```python
from build123d import *

# Parameters (mm, degrees)
SKETCH1_R          = 12.573
EXTRUDE1_DEPTH     = 2.1844
CUT_EXTRUDE1_DEPTH = 18.914582366
SKETCH4_R          = 4.6101
CUT_EXTRUDE2_DEPTH = 18.914582366
SKETCH5_R          = 0.508
CUT_EXTRUDE3_DEPTH = 18.914582366


with BuildPart() as part:
    # Sketch1 → Extrude1 (new body)
    with BuildSketch(Plane.XY):
        Circle(SKETCH1_R)
    extrude(amount=EXTRUDE1_DEPTH)

    # Sketch2 → Cut-Extrude1 (cut, through all)
    with BuildSketch(Plane.XY.offset(2.1844)):
        with BuildLine():
            Line((-7.159213379, 8.746626366), (-7.963619377, 9.729393373))
            ThreePointArc((-7.963619377, 9.729393373), (-8.89045356, 8.89045356), (-9.729393373, 7.963619377))
            Line((-9.729393373, 7.963619377), (-8.746626366, 7.159213379))
            ThreePointArc((-8.746626366, 7.159213379), (-9.076228299, 6.736459669), (-9.385415604, 6.298554036))
            Line((-9.385415604, 6.298554036), (-5.244666377, 3.907891355))
            ThreePointArc((-5.244666377, 3.907891355), (-4.624831902, 4.624831902), (-3.907891355, 5.244666377))
            Line((-3.907891355, 5.244666377), (-6.298554036, 9.385415604))
            ThreePointArc((-6.298554036, 9.385415604), (-6.736459669, 9.076228299), (-7.159213379, 8.746626366))
        make_face()
        with BuildLine():
            Line((-10.573373841, 3.995193941), (-11.761393373, 4.444092136))
            ThreePointArc((-11.761393373, 4.444092136), (-12.144585414, 3.254131854), (-12.407711513, 2.032))
            Line((-12.407711513, 2.032), (-11.15440732, 1.826747475))
            ThreePointArc((-11.15440732, 1.826747475), (-11.228474112, 1.295831056), (-11.277285356, 0.762))
            Line((-11.277285356, 0.762), (-6.495959994, 0.762))
            ThreePointArc((-6.495959994, 0.762), (-6.317637867, 1.692805964), (-6.006666377, 2.58806864))
            Line((-6.006666377, 2.58806864), (-10.147415604, 4.97873132))
            ThreePointArc((-10.147415604, 4.97873132), (-10.372059354, 4.492014443), (-10.573373841, 3.995193941))
        make_face()
        with BuildLine():
            Line((-11.15440732, -1.826747475), (-12.407711513, -2.032))
            ThreePointArc((-12.407711513, -2.032), (-12.144585414, -3.254131854), (-11.761393373, -4.444092136))
            Line((-11.761393373, -4.444092136), (-10.573373841, -3.995193941))
            ThreePointArc((-10.573373841, -3.995193941), (-10.372059354, -4.492014443), (-10.147415604, -4.97873132))
            Line((-10.147415604, -4.97873132), (-6.006666377, -2.58806864))
            ThreePointArc((-6.006666377, -2.58806864), (-6.317637867, -1.692805964), (-6.495959994, -0.762))
            Line((-6.495959994, -0.762), (-11.277285356, -0.762))
            ThreePointArc((-11.277285356, -0.762), (-11.228474112, -1.295831056), (-11.15440732, -1.826747475))
        make_face()
        with BuildLine():
            Line((-8.746626366, -7.159213379), (-9.729393373, -7.963619377))
            ThreePointArc((-9.729393373, -7.963619377), (-8.89045356, -8.89045356), (-7.963619377, -9.729393373))
            Line((-7.963619377, -9.729393373), (-7.159213379, -8.746626366))
            ThreePointArc((-7.159213379, -8.746626366), (-6.736459669, -9.076228299), (-6.298554036, -9.385415604))
            Line((-6.298554036, -9.385415604), (-3.907891355, -5.244666377))
            ThreePointArc((-3.907891355, -5.244666377), (-4.624831902, -4.624831902), (-5.244666377, -3.907891355))
            Line((-5.244666377, -3.907891355), (-9.385415604, -6.298554036))
            ThreePointArc((-9.385415604, -6.298554036), (-9.076228299, -6.736459669), (-8.746626366, -7.159213379))
        make_face()
        with BuildLine():
            ThreePointArc((-4.444092136, -11.761393373), (-3.254131854, -12.144585414), (-2.032, -12.407711513))
            Line((-2.032, -12.407711513), (-1.826747475, -11.15440732))
            ThreePointArc((-1.826747475, -11.15440732), (-1.295831056, -11.228474112), (-0.762, -11.277285356))
            Line((-0.762, -11.277285356), (-0.762, -6.495959994))
            ThreePointArc((-0.762, -6.495959994), (-1.692805964, -6.317637867), (-2.58806864, -6.006666377))
            Line((-2.58806864, -6.006666377), (-4.97873132, -10.147415604))
            ThreePointArc((-4.97873132, -10.147415604), (-4.492014443, -10.372059354), (-3.995193941, -10.573373841))
            Line((-3.995193941, -10.573373841), (-4.444092136, -11.761393373))
        make_face()
        with BuildLine():
            ThreePointArc((2.032, -12.407711513), (3.254131854, -12.144585414), (4.444092136, -11.761393373))
            Line((4.444092136, -11.761393373), (3.995193941, -10.573373841))
            ThreePointArc((3.995193941, -10.573373841), (4.492014443, -10.372059354), (4.97873132, -10.147415604))
            Line((4.97873132, -10.147415604), (2.58806864, -6.006666377))
            ThreePointArc((2.58806864, -6.006666377), (1.692805964, -6.317637867), (0.762, -6.495959994))
            Line((0.762, -6.495959994), (0.762, -11.277285356))
            ThreePointArc((0.762, -11.277285356), (1.295831056, -11.228474112), (1.826747475, -11.15440732))
            Line((1.826747475, -11.15440732), (2.032, -12.407711513))
        make_face()
        with BuildLine():
            ThreePointArc((7.963619377, -9.729393373), (8.89045356, -8.89045356), (9.729393373, -7.963619377))
            Line((9.729393373, -7.963619377), (8.746626366, -7.159213379))
            ThreePointArc((8.746626366, -7.159213379), (9.076228299, -6.736459669), (9.385415604, -6.298554036))
            Line((9.385415604, -6.298554036), (5.244666377, -3.907891355))
            ThreePointArc((5.244666377, -3.907891355), (4.624831902, -4.624831902), (3.907891355, -5.244666377))
            Line((3.907891355, -5.244666377), (6.298554036, -9.385415604))
            ThreePointArc((6.298554036, -9.385415604), (6.736459669, -9.076228299), (7.159213379, -8.746626366))
            Line((7.159213379, -8.746626366), (7.963619377, -9.729393373))
        make_face()
        with BuildLine():
            ThreePointArc((11.761393373, -4.444092136), (12.144585414, -3.254131854), (12.407711513, -2.032))
            Line((12.407711513, -2.032), (11.15440732, -1.826747475))
            ThreePointArc((11.15440732, -1.826747475), (11.228474112, -1.295831056), (11.277285356, -0.762))
            Line((11.277285356, -0.762), (6.495959994, -0.762))
            ThreePointArc((6.495959994, -0.762), (6.317637867, -1.692805964), (6.006666377, -2.58806864))
            Line((6.006666377, -2.58806864), (10.147415604, -4.97873132))
            ThreePointArc((10.147415604, -4.97873132), (10.372059354, -4.492014443), (10.573373841, -3.995193941))
            Line((10.573373841, -3.995193941), (11.761393373, -4.444092136))
        make_face()
        with BuildLine():
            ThreePointArc((12.407711513, 2.032), (12.144585414, 3.254131854), (11.761393373, 4.444092136))
            Line((11.761393373, 4.444092136), (10.573373841, 3.995193941))
            ThreePointArc((10.573373841, 3.995193941), (10.372059354, 4.492014443), (10.147415604, 4.97873132))
            Line((10.147415604, 4.97873132), (6.006666377, 2.58806864))
            ThreePointArc((6.006666377, 2.58806864), (6.317637867, 1.692805964), (6.495959994, 0.762))
            Line((6.495959994, 0.762), (11.277285356, 0.762))
            ThreePointArc((11.277285356, 0.762), (11.228474112, 1.295831056), (11.15440732, 1.826747475))
            Line((11.15440732, 1.826747475), (12.407711513, 2.032))
        make_face()
        with BuildLine():
            ThreePointArc((9.729393373, 7.963619377), (8.89045356, 8.89045356), (7.963619377, 9.729393373))
            Line((7.963619377, 9.729393373), (7.159213379, 8.746626366))
            ThreePointArc((7.159213379, 8.746626366), (6.736459669, 9.076228299), (6.298554036, 9.385415604))
            Line((6.298554036, 9.385415604), (3.907891355, 5.244666377))
            ThreePointArc((3.907891355, 5.244666377), (4.624831902, 4.624831902), (5.244666377, 3.907891355))
            Line((5.244666377, 3.907891355), (9.385415604, 6.298554036))
            ThreePointArc((9.385415604, 6.298554036), (9.076228299, 6.736459669), (8.746626366, 7.159213379))
            Line((8.746626366, 7.159213379), (9.729393373, 7.963619377))
        make_face()
        with BuildLine():
            ThreePointArc((4.97873132, 10.147415604), (4.492014443, 10.372059354), (3.995193941, 10.573373841))
            Line((3.995193941, 10.573373841), (4.444092136, 11.761393373))
            ThreePointArc((4.444092136, 11.761393373), (3.254131854, 12.144585414), (2.032, 12.407711513))
            Line((2.032, 12.407711513), (1.826747475, 11.15440732))
            ThreePointArc((1.826747475, 11.15440732), (1.295831056, 11.228474112), (0.762, 11.277285356))
            Line((0.762, 11.277285356), (0.762, 6.495959994))
            ThreePointArc((0.762, 6.495959994), (1.692805964, 6.317637867), (2.58806864, 6.006666377))
            Line((2.58806864, 6.006666377), (4.97873132, 10.147415604))
        make_face()
        with BuildLine():
            Line((-1.826747475, 11.15440732), (-2.032, 12.407711513))
            ThreePointArc((-2.032, 12.407711513), (-3.254131854, 12.144585414), (-4.444092136, 11.761393373))
            Line((-4.444092136, 11.761393373), (-3.995193941, 10.573373841))
            ThreePointArc((-3.995193941, 10.573373841), (-4.492014443, 10.372059354), (-4.97873132, 10.147415604))
            Line((-4.97873132, 10.147415604), (-2.58806864, 6.006666377))
            ThreePointArc((-2.58806864, 6.006666377), (-1.692805964, 6.317637867), (-0.762, 6.495959994))
            Line((-0.762, 6.495959994), (-0.762, 11.277285356))
            ThreePointArc((-0.762, 11.277285356), (-1.295831056, 11.228474112), (-1.826747475, 11.15440732))
        make_face()
    extrude(amount=-CUT_EXTRUDE1_DEPTH, mode=Mode.SUBTRACT)

    # Sketch4 → Cut-Extrude2 (cut, through all)
    with BuildSketch(Plane.XY.offset(2.1844)):
        Circle(SKETCH4_R)
    extrude(amount=-CUT_EXTRUDE2_DEPTH, mode=Mode.SUBTRACT)

    # Sketch5 → Cut-Extrude3 (cut, through all)
    with BuildSketch(Plane.XY.offset(2.1844)):
        with Locations((0, 4.6101)):
            Circle(SKETCH5_R)
    extrude(amount=-CUT_EXTRUDE3_DEPTH, mode=Mode.SUBTRACT)


solid = part.part
```
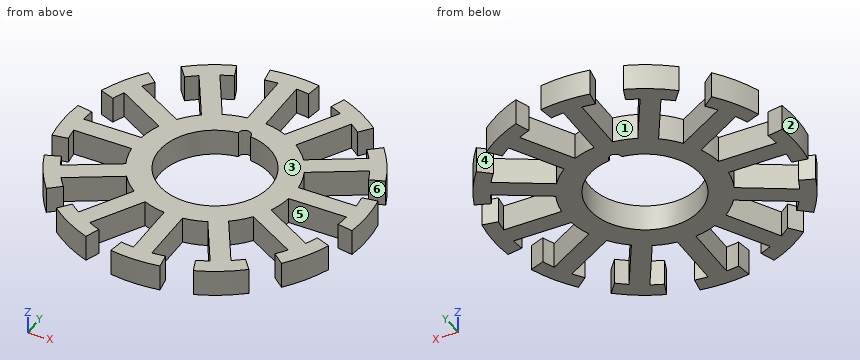
Design review of the part built by this model. Coordinates are the model's own, in mm. Face numbers are marked on the shaded views. A direction names the side the tool comes from. Coordinates: 2 decimals unless noted, no trailing zeros. Order: outer loops, then holes, each group sorted by start corner. A loop starts at its lowest first (then second) coordinate and runs counter-clockwise, first axis right, second up. Notation, with made-up numbers: (-27, 88.25) -> (5, 88.25) arc R12 ccw to (5, 102.25) -> close; hole circle Ø9 at (67, -26). An arc over 180 degrees is marked (long way). One line per item, written item: value. Start each with the question number.
Q1. Insertion check: pin 1 Ø5 at (x, y) = (-4, 0.5) entering from -Z; pin 2 Ø1 at (y, z) = (5, 0.5) entering from -X; pin 3 Ø0.7 at (y, z) = (8, 1.5) entering from -X; pin 4 Ø1 at (x, y) = (-3.5, -0.5) entering from +Z. Each pin has a flat end and moves straight along its axis. Give the tip position at first contact, or say it passes through.
Q2. Take a section at A-A, the plane y = 0. State the section outline as (x, z) points.
Q3. For probe 1 along Y at (x, z) = (0, 0.8); probe 2 along X at (y, z) = (0, 1.2); probe 3 along Y at (x, z) = (11.5, 1.8), list the stretches that pass through material, from the lowest coordinate up.
Q4. Mouldability with a two-part tool opening along X and no side actions: class the marked faces 1, 2 and 3 as pulls with the +X half, pulls with the -X half, needs draft (parallel to the pull), parting line crosses it, or undercut.
Q5. Tool access review of the marked faces 4, 5 and 6: name each direction out of +Z, -Z, +X, -X, +Y, -Y from which nothing blocks a thin tool from reaching the whole face with its end or side.
Q6. Take a section at B-B, the plane x = 0. State the section outline as (y, z) points.
Values follow:
1. pin 1: stops at z = 0
1. pin 2: stops at x = -11.74
1. pin 3: stops at x = -9.98
1. pin 4: passes through
2. outline: (-12.57, 0) -> (-4.61, 0) -> (-4.61, 2.18) -> (-12.57, 2.18) -> close; (4.61, 0) -> (12.57, 0) -> (12.57, 2.18) -> (4.61, 2.18) -> close
3. probe 1: y = -12.57 to -4.61, 5.12 to 12.57
3. probe 2: x = -12.57 to -4.61, 4.61 to 12.57
3. probe 3: y = -5.08 to -4.35, -1.88 to 1.88, 4.35 to 5.08
4. face 1: undercut
4. face 2: pulls with the -X half
4. face 3: needs draft
5. face 4: +Z, -Z, +Y
5. face 5: +Z, -Z
5. face 6: +Z, -Z, +X
6. outline: (-12.57, 0) -> (-4.61, 0) -> (-4.61, 2.18) -> (-12.57, 2.18) -> close; (5.12, 0) -> (12.57, 0) -> (12.57, 2.18) -> (5.12, 2.18) -> close
